Solid Edge part; units mm, degrees
sketch "Sketch1" plane through (0, 0, 0) normal (0, 0, 1) x (1, 0, 0)
  line L0 (-3.4648, -3.65) -> (88.4954, -3.65)
  line L1 (88.4954, -2.5) -> (88.4954, -3.65)
  line L2 (88.4954, -2.5) -> (90.9954, -2.5)
  line L3 (90.9954, 2.5) -> (88.4954, 2.5)
  line L4 (88.4954, 2.5) -> (88.4954, 3.65)
  line L5 (88.4954, 3.65) -> (-3.4648, 3.65)
  arc A0 (90.9954, 2.5) -> (90.9954, -2.5) centre (90.9954, 0) cw
  arc A1 (-3.4648, -3.65) -> (-3.4648, 3.65) centre (-6.5046, 0) cw
  circle A2 centre (90.9954, 0) radius 1
extrude "Protrusion1" add sketch "Sketch1" along normal blind 2
sketch "Sketch2" plane through (0, 0, 0) normal (0, 0, 1) x (1, 0, 0)
  arc A0 (8.113, -2.05) -> (8.113, 2.05) centre (8.1046, 0) ccw
  line L0 (8.113, 2.05) -> (-6.1019, 3.6277)
  arc A1 (-6.1019, 3.6277) -> (-6.1019, -3.6277) centre (-6.5046, 0) ccw
  line L1 (-6.1019, -3.6277) -> (8.113, -2.05)
extrude "Wycięcie_1" cut sketch "Sketch2" along normal blind 1.6
sketch "Sketch3" plane through (-0.55, 0, 1.6) normal (0, 0, -1) x (0.9939, -0.1103, 0)
  circle A0 centre (-5.9182, 0.6569) radius 1.925
extrude "Wyciągnięcie_2" add sketch "Sketch3" along normal mid plane 0.65
sketch "Sketch4" plane through (41.9756, 0, 0) normal (0, 0, -1) x (1, 0, 0)
  line L0 (-31.5172, 3.65) -> (-36.3172, 3.65)
  line L1 (-40.3172, 3.65) -> (-36.3172, 3.65)
  line L2 (-40.3172, 3.65) -> (-40.3172, -3.65)
  line L3 (-40.3172, -3.65) -> (-31.5172, -3.65)
  line L4 (-31.5172, -3.65) -> (-31.5172, 3.65)
extrude "Wyciągnięcie_4" add sketch "Sketch4" along normal blind 0.3
chamfer "Faza_3" [suppressed]
chamfer "Faza_2" [suppressed]
Verification items for the finished model (mm, model axes). A direction names the side the tool comes from. Give positions to 0.01 mm unless a question says otherwise; leave off trailing zeros. Loops run counter-clockwise (first coordinate to the right, second up) from the corner with the lowest first, then second, coordinate; pieces in that order, holes last.
1. Thickness scan on line 1 (X direction, y = 0.5, z = 0.7); line 2 (Z direction, x = 47, y = 2); line 3 (Y direction, x = 83.5, z = 1.3). Record the ranges inside material, lowest first.
2. Go/stop test with flat-tipped pins: pin 1 Ø0.6 at (y, z) = (3.5, 0.5) entering from +X; pin 2 Ø3 at (x, y) = (91, 0) entering from -Z; pin 3 Ø1 at (x, z) = (60.5, 1) entering from -Y. Record where each tip stops, or that it passes through.
3. Mould release check, pull along X, two halves, no side actions. Record for faces 1 (the flat face through (6, 0, 0)), 2 (the flat face through (-8, 4, 0)), 3 (the cylindrical face through (93.495, 0.055, 0.986)): released by +X, released by -X, zero draft, split by the parting line, or undercut.
4. Section check A-A, the plane z = 0.8. Enter the section's corners in (x, y).
5. Section check B-B, the plane x = 11.5. Enter the section's corners in (y, z), then the cut area to 3 significant figures.
6. Set-up check for faces 4 (the cylindrical face through (-10.154, -0.086, 0.789)), 5 (the flat face through (42, -3.65, 1)), 6 (the flat face through (90, 2.5, 1)): record each of +Z, -Z, +X, -X, +Y, -Y from which the full face is reachable in a straight line by a thin tool's end or side.
Geometry says:
1. line 1: x = -11.23 to -10.12, 10.09 to 90.13, 91.86 to 93.44
1. line 2: z = 0 to 2
1. line 3: y = -3.65 to 3.65
2. pin 1: stops at x = 88.5
2. pin 2: stops at z = 0
2. pin 3: stops at y = -3.65
3. face 1: undercut
3. face 2: zero draft
3. face 3: released by +X
4. outline: (-3.46, -3.65) - (88.5, -3.65) - (88.5, -2.5) - (91, -2.5) arc R2.5 ccw to (91, 2.5) - (88.5, 2.5) - (88.5, 3.65) - (-3.46, 3.65) arc R4.75 ccw (long way) to start; hole (-6.1, -3.63) - (8.11, -2.05) arc R2.05 ccw to (8.11, 2.05) - (-6.1, 3.63) arc R3.65 ccw (long way) to start; hole circle Ø2 at (91, 0)
5. outline: (-3.65, 0) - (3.65, 0) - (3.65, 2) - (-3.65, 2) - close
5. area: 14.6 mm2
6. face 4: -Z
6. face 5: +Z, -Z, +X, -Y
6. face 6: +Z, -Z, +X, +Y
